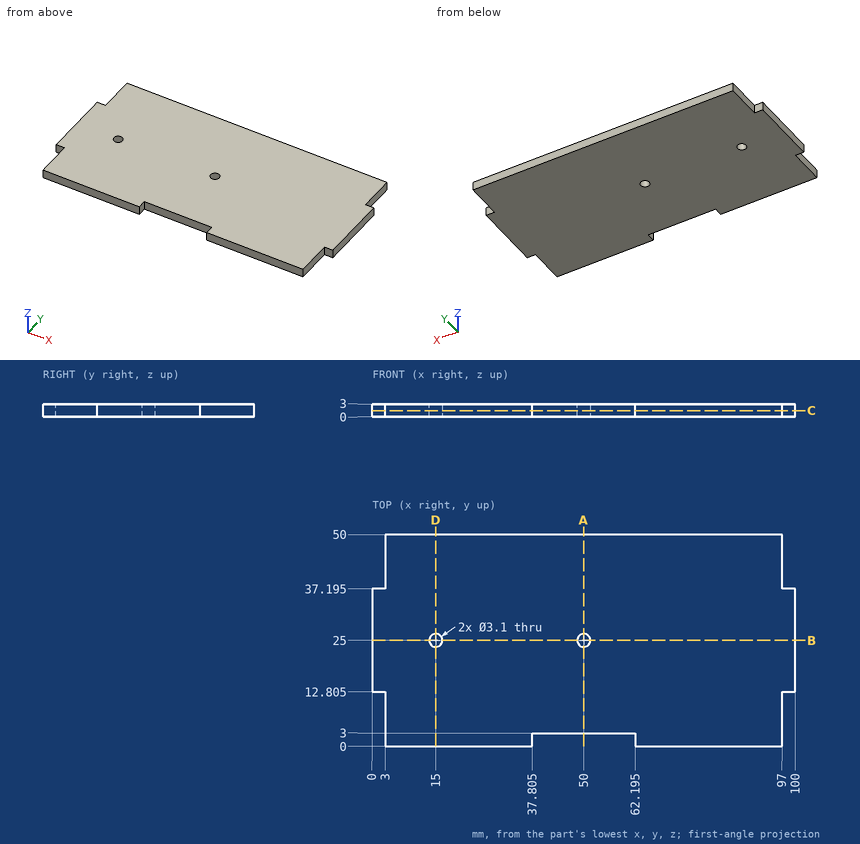
Input: dimensioned drawing with shaded views. Units: mm. Origin: part minimum x, y, z. Give positions to 0.01 mm unless a question says otherwise; leave off trailing zeros. Order: outer loops, then holes, each group sorted by start corner. A loop starts at its lowest first (then second) coordinate and runs counter-clockwise, first axis right, second up.
(1) Material intervals for line 1 along Y through (x, z) = (50, 1.65); line 2 along Y through (x, z) = (15, 0.8); line 3 along X through (y, z) = (24, 2.75), sorted ascending.
(2) Section query B-B (y = 25). Return the cut outline in (x, z).
(3) Contact query for flat-ended pins moving along their axis: P1, Ø1.5, axis at x = 2, z = 2, coming from the +Y side (3 decimals); P2, Ø0.9, axis at y = 45, z = 1, coming from the +X side; P3, Ø1.5, axis at x = 98.5, z = 1, coming from the -Y side (3 decimals). Output: stop coordinate, or through.
(4) Section query A-A (x = 50). Return the cut outline in (y, z).
(5) Section query D-D (x = 15). Return the cut outline in (y, z), plus the area to 3 significant figures.
(6) Section query C-C (z = 1.45). Return the cut outline in (x, y) (3 decimals).
Outcome:
1. line 1: y = 3 to 23.45, 26.55 to 50
1. line 2: y = 0 to 23.45, 26.55 to 50
1. line 3: x = 0 to 13.82, 16.18 to 48.82, 51.18 to 100
2. outline: (0, 0) - (13.45, 0) - (13.45, 3) - (0, 3) - close; (16.55, 0) - (48.45, 0) - (48.45, 3) - (16.55, 3) - close; (51.55, 0) - (100, 0) - (100, 3) - (51.55, 3) - close
3. P1: stops at y = 37.195
3. P2: stops at x = 97
3. P3: stops at y = 12.805
4. outline: (3, 0) - (23.45, 0) - (23.45, 3) - (3, 3) - close; (26.55, 0) - (50, 0) - (50, 3) - (26.55, 3) - close
5. outline: (0, 0) - (23.45, 0) - (23.45, 3) - (0, 3) - close; (26.55, 0) - (50, 0) - (50, 3) - (26.55, 3) - close
5. area: 141 mm2
6. outline: (0, 12.805) - (3, 12.805) - (3, 0) - (37.805, 0) - (37.805, 3) - (62.195, 3) - (62.195, 0) - (97, 0) - (97, 12.805) - (100, 12.805) - (100, 37.195) - (97, 37.195) - (97, 50) - (3, 50) - (3, 37.195) - (0, 37.195) - close; hole circle Ø3.1 at (15, 25); hole circle Ø3.1 at (50, 25)
